Check sheet for the modelled part. Datum: model origin and axes. Units: mm. Face numbers are marked on the shaded views. A direction names the side the tool comes from. Give positions to 0.01 mm unless a question says otherwise; leave off trailing zeros. Loops run counter-clockwise (first coordinate to the right, second up) from the corner with the lowest first, then second, coordinate; pieces in that order, holes last. Notation, with made-up numbers: M -6.5,-0.5 L 31.5,-0.5 A19 cw 31.5,9.5 Z; hole C -37.5,72 d3. An arc over 180 degrees is marked long. Write each question's results on one line, items separated by ' | '. Start each with the question number.
1. Tool access check on the marked faces 4, 5 and 6. Record the directions out of +Z, -Z, +X, -X, +Y, -Y that give a thin tool (end or side, any length) a straight path to the whole face; none if there is none.
2. Go/stop test with flat-tipped pins: pin 1 (1 mm diameter, centred on y = -36.5, z = 17, fed in from -X); pin 2 (7.5 mm diameter, centred on x = -13.5, y = -35.5, fed in from +Z). Record where each tip stops, or that it passes through.
3. Sectioned sample at C-C on x = -16. Record the cut outline in (y, z), and give its area (3 significant figures).
4. Sectioned sample at D-D on z = 67. Record the cut outline in (x, y).
5. Material ranges on line 1 along Z through (x, y) = (-16, -51.75); line 2 along Z through (x, y) = (-13.75, -42.5); line 3 along Z through (x, y) = (-10.25, -57), recorded low to high.
6. Sectioned sample at B-B on y = -5. Record the cut outline in (x, z), and give its area (3 significant figures).
7. Sectioned sample at A-A on z = 35. Record the cut outline in (x, y).
8. Draft check along Z on the marked faces 1, 2 and 3. Enter one of: pulls with the +Z half, pulls with the -Z half, needs draft (parallel to the pull), parting line crosses it, or undercut.
```python
from build123d import *

# Parameters (mm, degrees)
F0_R     = 3.2
F1_DEPTH = 60
F2_W     = 23.016388
F2_H     = 20
F3_DEPTH = 72.501
F4_W     = 17
F4_H     = 60
F5_DEPTH = 50
F6_R     = 3
F7_DEPTH = 25


with BuildPart() as f1:
    # F0 (on Front) → F1 (new body)
    with BuildSketch(Plane.XZ):
        with BuildLine():
            Line((-10, 64), (-10, 0))
            Line((-10, 0), (0, 0))
            Line((0, 0), (0, 70))
            Line((0, 70), (-11.390228, 70))
            ThreePointArc((-11.390228, 70), (-21.5, 67), (-11.390228, 64))
            Line((-11.390228, 64), (-10, 64))
        make_face()
        with Locations((-16, 67)):
            Circle(F0_R, mode=Mode.SUBTRACT)
    extrude(amount=F1_DEPTH)

    # F2 (on Top) → F3 (cut, through all)
    with BuildSketch(Plane.XY):
        with Locations((-21.508194, -30)):
            Rectangle(F2_W, F2_H)
    extrude(amount=F3_DEPTH, mode=Mode.SUBTRACT)

    # F4 (on Top) → F5 (join)
    with BuildSketch(Plane.XY):
        with Locations((-8.5, -30)):
            Rectangle(F4_W, F4_H)
    extrude(amount=F5_DEPTH)

    # F6 (on face) → F7 (cut)
    with BuildSketch(Plane.YZ):
        with Locations((-44.56006, 35)):
            Circle(F6_R)
        with BuildLine():
            ThreePointArc((-18.885411, 43.756471), (-17.460533, 33.783836), (-19.772981, 23.978923))
            ThreePointArc((-19.772981, 23.978923), (-18.314924, 20.18622), (-14.52222, 21.644278))
            ThreePointArc((-14.52222, 21.644278), (-11.719915, 33.52621), (-13.446631, 45.611395))
            ThreePointArc((-13.446631, 45.611395), (-17.093483, 47.403323), (-18.885411, 43.756471))
        make_face()
    extrude(amount=-F7_DEPTH, mode=Mode.SUBTRACT)


solid = f1.part
```
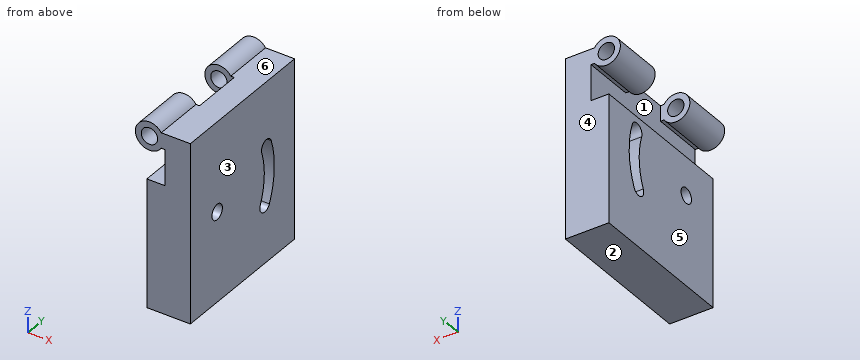
Output values:
1) face 4: +Z, -Z, +X, -X, +Y | face 5: -Z, -X, +Y, -Y | face 6: +Z, +X, +Y, -Y
2) pin 1: x = -17 | pin 2: z = 70
3) outline: M -60,0 L 0,0 L 0,50 L -60,50 Z; M -60,61.5 L -40,61.5 L -40,63.8 L -60,63.8 Z; M -60,70.2 L -40,70.2 L -40,72.5 L -60,72.5 Z; M -20,61.5 L 0,61.5 L 0,63.8 L -20,63.8 Z; M -20,70.2 L 0,70.2 L 0,72.5 L -20,72.5 Z; hole C -44.56,35 d6; hole M -19.77,23.98 A2.87 ccw -14.52,21.64 A32.87 ccw -13.45,45.61 A2.87 ccw -18.89,43.76 A27.13 cw Z | area: 3,000 mm2
4) outline: M -21.5,-60 L -19.2,-60 L -19.2,-40 L -21.5,-40 Z; M -21.5,-20 L -19.2,-20 L -19.2,0 L -21.5,0 Z; M -12.8,-60 L 0,-60 L 0,0 L -12.8,0 L -12.8,-20 L -10,-20 L -10,-40 L -12.8,-40 Z
5) line 1: 0 to 50, 61.5 to 63.8, 70.2 to 72.5 | line 2: 0 to 32.82, 37.18 to 50, 61.98 to 64.72, 69.28 to 72.02 | line 3: 0 to 50, 64 to 70
6) outline: M -17,0 L 0,0 L 0,70 L -11.39,70 A5.5 ccw long -11.39,64 L -10,64 L -10,50 L -17,50 Z; hole C -16,67 d6.4 | area: 1,120 mm2
7) outline: M -17,-60 L 0,-60 L 0,-47.56 L -17,-47.56 Z; M -17,-41.56 L 0,-41.56 L 0,-17.43 L -17,-17.43 Z; M -17,-11.69 L 0,-11.69 L 0,0 L -17,0 Z
8) face 1: undercut | face 2: pulls with the -Z half | face 3: needs draft
